from build123d import *

# Parameters (mm, degrees)
SKETCH1_R           = 5
BOSS_EXTRUDE1_DEPTH = 20
FILLET1_R           = 1
CUT_EXTRUDE1_DEPTH  = 15
SKETCH4_R           = 3.05
CUT_EXTRUDE2_DEPTH  = 3


with BuildPart() as part:
    # Sketch1 → Boss-Extrude1 (new body)
    with BuildSketch(Plane(origin=(0, 0, 0), x_dir=(1, 0, 0), z_dir=(0, 1, 0))):
        with Locations(Location((0, 0, 0), (0, 0, 270))):
            Circle(SKETCH1_R)
    extrude(amount=BOSS_EXTRUDE1_DEPTH)

    # Fillet1
    fillet1_edges = [part.edges().sort_by_distance(p)[0] for p in [
        (0, 20, -5),
    ]]
    fillet(fillet1_edges, radius=FILLET1_R)

    # Sketch2 → Cut-Extrude1 (cut)
    with BuildSketch(Plane(origin=(0, 0, 0), x_dir=(-1, 0, 0), z_dir=(0, -1, 0))):
        with BuildLine():
            ThreePointArc((1.44, 2.688661377), (-3.05, 0), (1.44, -2.688661377))
            Line((1.44, -2.688661377), (1.44, 2.688661377))
        make_face()
    extrude(amount=-CUT_EXTRUDE1_DEPTH, mode=Mode.SUBTRACT)

    # Sketch4 → Cut-Extrude2 (cut)
    with BuildSketch(Plane(origin=(0, 0, 0), x_dir=(-1, 0, 0), z_dir=(0, -1, 0))):
        with Locations(Location((0, 0, 0), (0, 0, 90))):
            Circle(SKETCH4_R)
    extrude(amount=-CUT_EXTRUDE2_DEPTH, mode=Mode.SUBTRACT)


solid = part.part
The listing builds one solid part. Answer for the finished solid, in the listing's coordinates (mm). A direction names the side the tool comes from. Coordinates: 2 decimals unless noted, no trailing zeros. Write each loop counter-clockwise with the first axis right and the second up, starting at its lowest first coordinate (ties: lowest second). Pieces come first, ordered by that corner, then holes. Notation, with made-up numbers: (79.25, 16) -> (106.25, 16) arc R32 cw to (106.25, 45) -> close; hole circle Ø7 at (84.5, 45.25). An arc over 180 degrees is marked (long way). One line per question, with ' | ' between items.
1. Which of the six approach directions +Z, -Z, +X, -X, +Y, -Y give full straight-line access (tool end or side, diameter ignored) to faces 1 (the flat face through (-1.44, 9, 0)), 2 (the flat face through (0, 20, 0))?
Verdict:
face 1: -Y | face 2: +Z, -Z, +X, -X, +Y
2. Section C-C (y = 11) is taken. Determine the outline of the cut face in (x, z), and give its area (3 significant figures).
Verdict:
outline: circle Ø10 at (0, 0); hole (-1.44, -2.69) arc R3.05 ccw (long way) to (-1.44, 2.69) -> close | area: 55.5 mm^2
3. Straight lines are drawn through the part: line 1 (X direction, y = 7.5, z = 0); line 2 (Y direction, x = -0.5, z = -2); line 3 (Y direction, x = -2, z = 1.75). For each, find the intervals that lie inside material, in ascending order.
Verdict:
line 1: x = -5 to -1.44, 3.05 to 5 | line 2: y = 15 to 20 | line 3: y = 3 to 20
4. Section B-B (z = 0) is taken. Determine the outline of the cut face in (x, y), and give its area (3 significant figures).
Verdict:
outline: (-5, 0) -> (-3.05, 0) -> (-3.05, 3) -> (-1.44, 3) -> (-1.44, 15) -> (3.05, 15) -> (3.05, 0) -> (5, 0) -> (5, 19) arc R1 ccw to (4, 20) -> (-4, 20) arc R1 ccw to (-5, 19) -> close | area: 127 mm^2
5. For a pull along Z with two mould halves and no side action, classify faces 3 (the cylindrical face through (-4.88, 9.37, -1.08)), 4 (the flat face through (-2, 3, 0)), 5 (the flat face through (-3.3, 0, -0.1)), 6 (the flat face through (0, 15, 0)) as released by +Z, released by -Z, zero draft, split by the parting line, or undercut.
Verdict:
face 3: split by the parting line | face 4: undercut | face 5: zero draft | face 6: undercut
6. Given pin 1 Ø1.3 at (x, z) = (0.5, 1.5) entering from -Y; pin 2 Ø1.5 at (y, z) = (2, -4) entering from -X; pin 3 Ø1.5 at (x, y) = (1, 16.5) entering from +Z, each flat-ended and moving along its own axis, determine where each tip first touches the part or whether it passes through.
Verdict:
pin 1: stops at y = 15 | pin 2: stops at x = -3.8 | pin 3: stops at z = 4.99
7. Section A-A (x = 0) is taken. Determine the outline of the cut face in (y, z), and give its area (3 significant figures).
Verdict:
outline: (0, -5) -> (19, -5) arc R1 ccw to (20, -4) -> (20, 4) arc R1 ccw to (19, 5) -> (0, 5) -> (0, 3.05) -> (15, 3.05) -> (15, -3.05) -> (0, -3.05) -> close | area: 108 mm^2
8. Section D-D (y = 16.25) is taken. Determine the outline of the cut face in (x, z), and give its area (3 significant figures).
Verdict:
outline: circle Ø10 at (0, 0) | area: 78.5 mm^2
